from build123d import *

# Parameters (mm, degrees)
ESQUISSE3_R             = 6.15
ESQUISSE3_R_2           = 1.65
BOSS_EXTRU_2_DEPTH      = 3.5
ESQUISSE4_R             = 18.65
BOSS_EXTRU_3_DEPTH      = 23.2
ESQUISSE5_R             = 2.05
ENL_V_MAT_EXTRU_1_DEPTH = 31


with BuildPart() as part:
    # Esquisse3 → Boss.-Extru.2 (new body)
    with BuildSketch(Plane.XY):
        with BuildLine():
            Line((-20, 0), (-20, -17))
            ThreePointArc((-20, -17), (-20.292893219, -17.707106781), (-21, -18))
            Line((-21, -18), (-30, -18))
            Line((-30, -18), (-30, -23))
            Line((-30, -23), (30, -23))
            Line((30, -23), (30, -18))
            Line((30, -18), (21, -18))
            ThreePointArc((21, -18), (20.292893219, -17.707106781), (20, -17))
            Line((20, -17), (20, 0))
            ThreePointArc((20, 0), (0, 20), (-20, 0))
        make_face()
        with Locations((0, -7)):
            Circle(ESQUISSE3_R, mode=Mode.SUBTRACT)
        with Locations((-15.5, 0)):
            Circle(ESQUISSE3_R_2, mode=Mode.SUBTRACT)
        with Locations((-7.75, 13.423393759)):
            Circle(ESQUISSE3_R_2, mode=Mode.SUBTRACT)
        with Locations((7.75, 13.423393759)):
            Circle(ESQUISSE3_R_2, mode=Mode.SUBTRACT)
        with Locations((15.5, 0)):
            Circle(ESQUISSE3_R_2, mode=Mode.SUBTRACT)
        with Locations((7.75, -13.423393759)):
            Circle(ESQUISSE3_R_2, mode=Mode.SUBTRACT)
        with Locations((-7.75, -13.423393759)):
            Circle(ESQUISSE3_R_2, mode=Mode.SUBTRACT)
    extrude(amount=-BOSS_EXTRU_2_DEPTH)

    # Esquisse4 → Boss.-Extru.3 (add)
    with BuildSketch(Plane(origin=(0, 0, -3.5), x_dir=(-1, 0, 0), z_dir=(0, 0, -1))):
        with BuildLine():
            Line((-20, 0), (-20, -17))
            ThreePointArc((-20, -17), (-20.292893219, -17.707106781), (-21, -18))
            Line((-21, -18), (-30, -18))
            Line((-30, -18), (-30, -23))
            Line((-30, -23), (30, -23))
            Line((30, -23), (30, -18))
            Line((30, -18), (21, -18))
            ThreePointArc((21, -18), (20.292893219, -17.707106781), (20, -17))
            Line((20, -17), (20, 0))
            ThreePointArc((20, 0), (0, 20), (-20, 0))
        make_face()
        Circle(ESQUISSE4_R, mode=Mode.SUBTRACT)
    extrude(amount=BOSS_EXTRU_3_DEPTH)

    # Esquisse5 → Enlèv. mat.-Extru.1 (cut)
    with BuildSketch(Plane(origin=(0, 0, 0), x_dir=(1, 0, 0), z_dir=(0, 1, 0))):
        with Locations(Location((-25.5, 21.7, 0), (0, 0, 270))):
            Circle(ESQUISSE5_R)
        with Locations(Location((-25.5, 5, 0), (0, 0, 270))):
            Circle(ESQUISSE5_R)
        with Locations(Location((25.5, 5, 0), (0, 0, 270))):
            Circle(ESQUISSE5_R)
        with Locations(Location((25.5, 21.7, 0), (0, 0, 270))):
            Circle(ESQUISSE5_R)
    extrude(amount=-ENL_V_MAT_EXTRU_1_DEPTH, mode=Mode.SUBTRACT)


solid = part.part
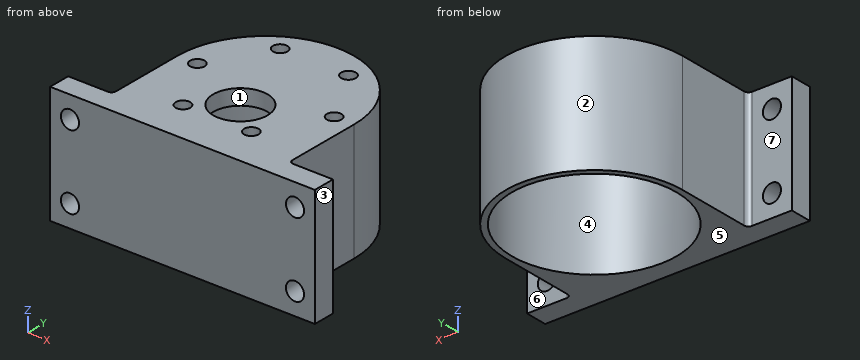
Check sheet for the modelled part. Datum: model origin and axes. Units: mm. Face numbers are marked on the shaded views. A direction names the side the tool comes from. Round coordinates to 2 decimals unless told otherwise and drop trailing zeros. Loops run counter-clockwise (first coordinate to the right, second up) from the corner with the lowest first, then second, coordinate; pieces in that order, holes last. Notation, with made-up numbers: (47, -8) - (82, -8) arc R31 cw to (82, 24) - close; hole circle Ø1 at (-5, 78). An arc over 180 degrees is marked (long way). Answer as CSV lines item,"result". Start each with the question number.
Item 1: Section check C-C (y = -12.5). Record the boundary of the cut face in (x, z), and give its area (3 significant figures).
Item 2: Depth check by flat-ended pin: P1, Ø5.5, axis at x = 7.75, y = 13.42, coming from the -Z side; P2, Ø3, axis at y = 11, z = -17, coming from the -X side; P3, Ø8.5, axis at y = -11, z = -18.5, coming from the -X side; P4, Ø4, axis at x = -11.5, y = -13, coming from the -Z side. Enter the tip coordinate at first touch or a pass-through.
Item 3: Section check B-B (x = -25.5). Record the boundary of the cut face in (y, z).
Item 4: Set-up check for the marked faces 5, 6 and 7: record each of +Z, -Z, +X, -X, +Y, -Y from which the full face is reachable in a straight line by a thin tool's end or side.
Item 5: Section check D-D (x = -3). Record the boundary of the cut face in (y, z), and give its area (3 significant figures).
Item 6: Scan lines: line 1 (Y direction, x = -7.75, z = -1.3); line 2 (Z direction, x = 25, y = -21); line 3 (X direction, y = -20.6, z = -5). Record each from-to range of solid material in increasing order. Write a range as [from, to].
Item 7: Section check A-A (z = -21.7). Record the boundary of the cut face in (x, y), and give its area (3 significant figures).
Item 8: Release check for a two-part mould opening along X. For the marked faces 1, 2, 3 and 4 record: +X half, -X half, draft (parallel to the pull), parting line (faces both ways), or undercut.
Report:
1,outline,"(-20, -26.7) - (-13.84, -26.7) - (-13.84, -3.5) - (-9.12, -3.5) - (-9.12, 0) - (-20, 0) - close; (-6.38, -3.5) - (-2.75, -3.5) - (-2.75, 0) - (-6.38, 0) - close; (2.75, -3.5) - (6.38, -3.5) - (6.38, 0) - (2.75, 0) - close; (9.12, -3.5) - (13.84, -3.5) - (13.84, -26.7) - (20, -26.7) - (20, 0) - (9.12, 0) - close"
1,area,"387 mm2"
2,P1,"stops at z = -3.5"
2,P2,"stops at x = -17.6"
2,P3,"stops at x = -20"
2,P4,"stops at z = -26.7"
3,outline,"(-23, -26.7) - (-18, -26.7) - (-18, -23.75) - (-23, -23.75) - close; (-23, -19.65) - (-18, -19.65) - (-18, -7.05) - (-23, -7.05) - close; (-23, -2.95) - (-18, -2.95) - (-18, 0) - (-23, 0) - close"
4,face 5,"-Z, +X, -X, +Y, -Y"
4,face 6,"+Z, -Z, +X, +Y"
4,face 7,"+Z, -Z, -X, +Y"
5,outline,"(-23, -26.7) - (-18.41, -26.7) - (-18.41, -3.5) - (-12.37, -3.5) - (-12.37, 0) - (-23, 0) - close; (-1.63, -3.5) - (18.41, -3.5) - (18.41, -26.7) - (19.77, -26.7) - (19.77, 0) - (-1.63, 0) - close"
5,area,"250 mm2"
6,line 1,"y = [-23, -15.07], [-11.77, 11.77], [15.07, 18.44]"
6,line 2,"z = [-26.7, -23.69], [-19.71, -6.99], [-3.01, 0]"
6,line 3,"x = [-30, -27.55], [-23.45, 23.45], [27.55, 30]"
7,outline,"(-30, -23) - (-27.55, -23) - (-27.55, -18) - (-30, -18) - close; (-23.45, -23) - (23.45, -23) - (23.45, -18) - (21, -18) arc R1 cw to (20, -17) - (20, 0) arc R20 ccw to (-20, 0) - (-20, -17) arc R1 cw to (-21, -18) - (-23.45, -18) - close; (27.55, -23) - (30, -23) - (30, -18) - (27.55, -18) - close; hole circle Ø37.3 at (0, 0)"
7,area,"515 mm2"
8,face 1,"undercut"
8,face 2,"parting line"
8,face 3,"+X half"
8,face 4,"undercut"
